Check sheet for the drawn part. Datum: minimum x, y, z corner. Units: mm. Round coordinates to 2 decimals unless told otherwise and drop trailing zeros. Write each loop counter-clockwise with the first axis right and the second up, starting at its lowest first coordinate (ties: lowest second). Pieces come first, ordered by that corner, then holes. Notation, with made-up numbers: M -28.75,-6.75 L -6.75,-6.75 A10 cw -6.75,2.25 Z; hole C -19.75,-4.5 d10. An arc over 180 degrees is marked long. Use a Markdown table: item, result.
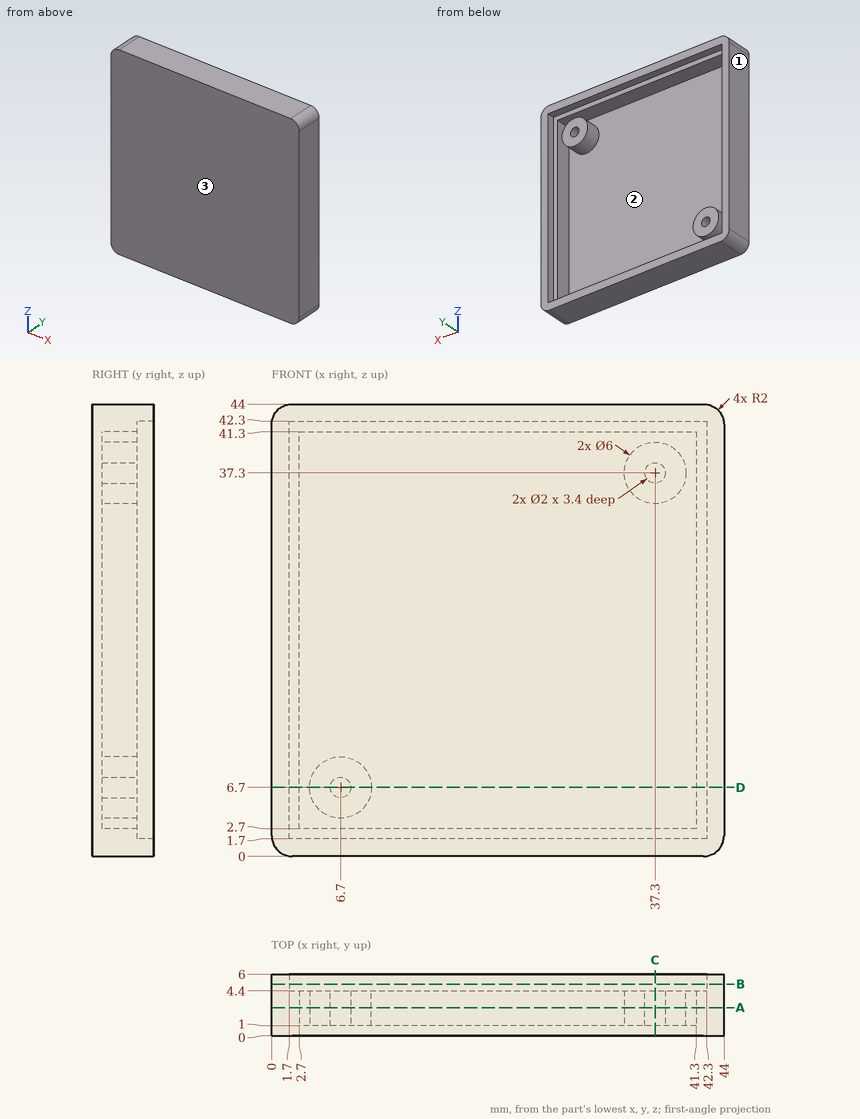
Item 1: Mould release check, pull along X, two halves, no side actions. Record for the marked faces 1, 2 and 3: +X half, -X half, draft (parallel to the pull), parting line (faces both ways), or undercut.
Outcome:
| item | result |
|---|---|
| face 1 | -X half |
| face 2 | undercut |
| face 3 | draft |
Item 2: Cross-section at A-A, the plane y = 2.75. Record the cut outline in (x, z).
Outcome:
| item | result |
|---|---|
| outline | M 0,2 A2 ccw 2,0 L 42,0 A2 ccw 44,2 L 44,42 A2 ccw 42,44 L 2,44 A2 ccw 0,42 Z; C 6.7,6.7 d6; C 37.3,37.3 d6; hole M 2.7,2.7 L 41.3,2.7 L 41.3,41.3 L 2.7,41.3 Z; hole C 6.7,6.7 d2; hole C 37.3,37.3 d2 |
Item 3: Cross-section at B-B, the plane y = 5.05. Record the cut outline in (x, z), and give its area (3 significant figures).
Outcome:
| item | result |
|---|---|
| outline | M 0,2 A2 ccw 2,0 L 42,0 A2 ccw 44,2 L 44,42 A2 ccw 42,44 L 2,44 A2 ccw 0,42 Z; hole M 1.7,1.7 L 42.3,1.7 L 42.3,42.3 L 1.7,42.3 Z |
| area | 284 mm2 |
Item 4: Cross-section at C-C, the plane x = 37.3. Record the cut outline in (y, z).
Outcome:
| item | result |
|---|---|
| outline | M 0,0 L 6,0 L 6,1.7 L 4.4,1.7 L 4.4,2.7 L 1,2.7 L 1,34.3 L 4.4,34.3 L 4.4,36.3 L 1,36.3 L 1,38.3 L 4.4,38.3 L 4.4,40.3 L 1,40.3 L 1,41.3 L 4.4,41.3 L 4.4,42.3 L 6,42.3 L 6,44 L 0,44 Z |
Item 5: Go/stop test with flat-tipped pins: pin 1 (5 mm diameter, centred on x = 38.5, z = 38, fed in from +Y); pin 2 (0.6 mm diameter, centred on x = 37, z = 37.5, fed in from +Y). Record where each tip stops, or that it passes through.
Outcome:
| item | result |
|---|---|
| pin 1 | stops at y = 4.4 |
| pin 2 | stops at y = 1 |
Item 6: Material ranges on line 1 along X through (y, z) = (2.4, 37.3); line 2 along Z through (x, y) = (37.5, 4.95), recorded low to high. Write a range as from..to.
Outcome:
| item | result |
|---|---|
| line 1 | x = 0..2.7, 34.3..36.3, 38.3..40.3, 41.3..44 |
| line 2 | z = 0..1.7, 42.3..44 |
Item 7: Cross-section at D-D, the plane z = 6.7. Record the cut outline in (x, y), and give its area (3 significant figures).
Outcome:
| item | result |
|---|---|
| outline | M 0,0 L 44,0 L 44,6 L 42.3,6 L 42.3,4.4 L 41.3,4.4 L 41.3,1 L 9.7,1 L 9.7,4.4 L 7.7,4.4 L 7.7,1 L 5.7,1 L 5.7,4.4 L 3.7,4.4 L 3.7,1 L 2.7,1 L 2.7,4.4 L 1.7,4.4 L 1.7,6 L 0,6 Z |
| area | 81.4 mm2 |
